from build123d import *

# Parameters (mm, degrees)
SKETCH_1_R          = 10
EXTRUDE_1_DEPTH     = 5
SKETCH_2_R          = 7.5
EXTRUDE_2_DEPTH     = 7
SKETCH_3_R          = 2.5
CUT_EXTRUDE_1_DEPTH = 12


with BuildPart() as part:
    # 草图1 → 凸台-拉伸1 (new body)
    with BuildSketch(Plane(origin=(0, 0, 0), x_dir=(1, 0, 0), z_dir=(0, 1, 0))):
        with Locations(Location((0, 0, 0), (0, 0, 270))):
            Circle(SKETCH_1_R)
    extrude(amount=EXTRUDE_1_DEPTH)

    # 草图2 → 凸台-拉伸2 (add)
    with BuildSketch(Plane(origin=(0, 5, 0), x_dir=(1, 0, 0), z_dir=(0, 1, 0))):
        with Locations(Location((0, 0, 0), (0, 0, 270))):
            Circle(SKETCH_2_R)
    extrude(amount=EXTRUDE_2_DEPTH)

    # 草图3 → 切除-拉伸1 (cut)
    with BuildSketch(Plane.XZ):
        with Locations(Location((0, 0, 0), (0, 0, 270))):
            Circle(SKETCH_3_R)
    extrude(amount=-CUT_EXTRUDE_1_DEPTH, mode=Mode.SUBTRACT)


solid = part.part
Geometry: final body of the model. Coordinates: model frame, mm. Coordinates: 2 decimals unless noted, no trailing zeros. Order: outer loops, then holes, each group sorted by start corner. A loop starts at its lowest first (then second) coordinate and runs counter-clockwise, first axis right, second up.
(1) Section query B-B (z = 0). Return the cut outline in (x, y), plus the area to 3 significant figures.
(2) Section query D-D (z = -6.75). Return the cut outline in (x, y), plus the area to 3 significant figures.
(3) Draft query along Z for faces 1 (the face through (7, 5, 4)), 2 (the face through (-2.44, 5.92, 0.54)), 3 (the face through (0.33, 8.451, -7.493)). Return one class per face: pulls with the +Z half, pulls with the -Z half, needs draft (parallel to the pull), parting line crosses it, or undercut.
(4) First-contact query: pin 1 (8 mm diameter, centred on x = 2, z = 1, fed in from -Y); pin 2 (4 mm diameter, centred on y = 8.5, z = 3.5, fed in from -X); pin 3 (4 mm diameter, centred on x = -3, y = 6, fed in from +Z); pin 4 (4 mm diameter, centred on y = 8, z = -6, fed in from -X). Flat tips, straight axial feed; report the tip coordinate or a pass-through.
(5) Material intervals for probe 1 along X at (y, z) = (9.5, 0); probe 2 along Y at (x, z) = (9.25, 2); probe 3 along Z at (x, y) = (1.5, 6.25), sorted ascending.
(6) Section query C-C (y = 3.75). Return the cut outline in (x, z), plus the area to 3 significant figures.
(7) Section query A-A (x = 0). Return the cut outline in (y, z), plus the area to 3 significant figures.
Solution:
1. outline: (-10, 0) - (-2.5, 0) - (-2.5, 12) - (-7.5, 12) - (-7.5, 5) - (-10, 5) - close; (2.5, 0) - (10, 0) - (10, 5) - (7.5, 5) - (7.5, 12) - (2.5, 12) - close
1. area: 145 mm2
2. outline: (-7.38, 0) - (7.38, 0) - (7.38, 5) - (3.27, 5) - (3.27, 12) - (-3.27, 12) - (-3.27, 5) - (-7.38, 5) - close
2. area: 120 mm2
3. face 1: needs draft
3. face 2: undercut
3. face 3: parting line crosses it
4. pin 1: stops at y = 0
4. pin 2: stops at x = -7.35
4. pin 3: stops at z = 9.92
4. pin 4: stops at x = -6.34
5. probe 1: x = -7.5 to -2.5, 2.5 to 7.5
5. probe 2: y = 0 to 5
5. probe 3: z = -7.35 to -2, 2 to 7.35
6. outline: circle Ø20 at (0, 0); hole circle Ø5 at (0, 0)
6. area: 295 mm2
7. outline: (0, -10) - (5, -10) - (5, -7.5) - (12, -7.5) - (12, -2.5) - (0, -2.5) - close; (0, 2.5) - (12, 2.5) - (12, 7.5) - (5, 7.5) - (5, 10) - (0, 10) - close
7. area: 145 mm2
